Source: three-view drawing plus pictorial views. Frame: mm from the lowest corner of the part. Coordinates: 2 decimals unless noted, no trailing zeros. Write each loop counter-clockwise with the first axis right and the second up, starting at its lowest first coordinate (ties: lowest second). Pieces come first, ordered by that corner, then holes. Notation, with made-up numbers: (-21.5, 56.25) - (-11.5, 56.25) arc R23 ccw to (-11.5, 82.25) - close; hole circle Ø4 at (-22.75, 50.5). An arc over 180 degrees is marked (long way). One line per item, written item: value.
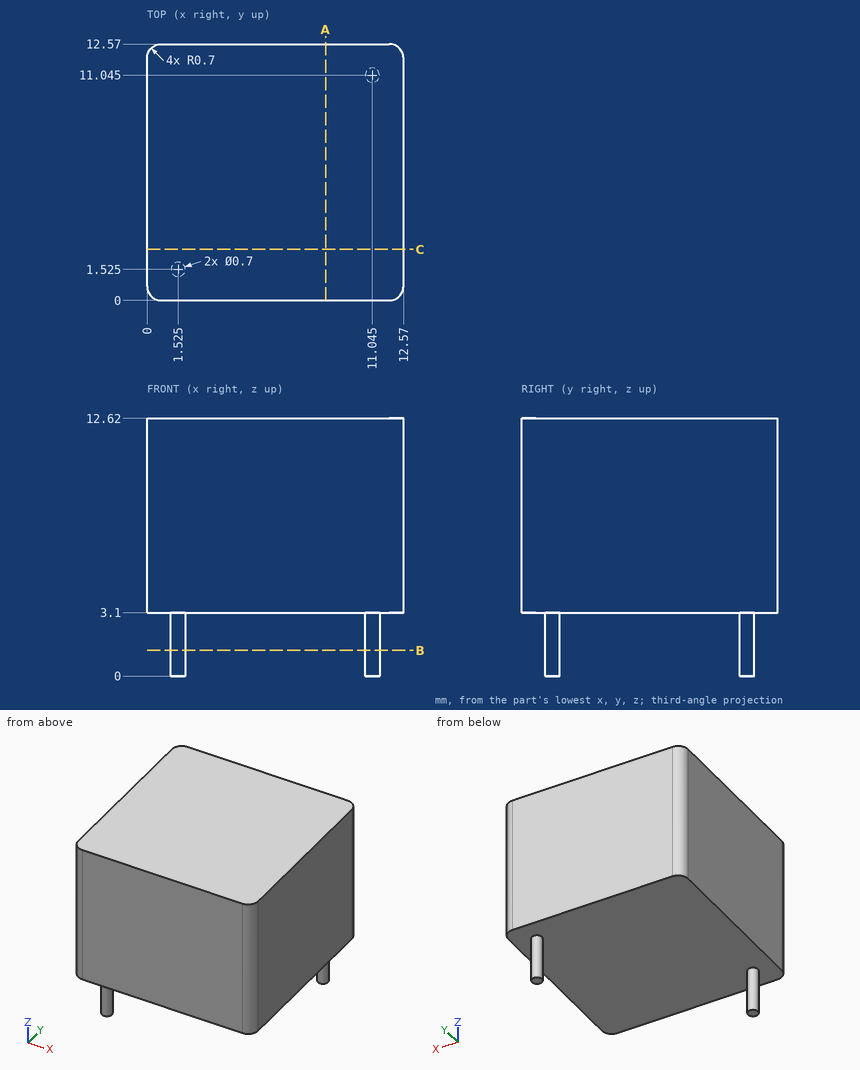
1) Section query B-B on z = 1.25. Output: boundary loops of the cut face in (x, y) (3 decimals), then the cut area to 3 significant figures.
Values found:
outline: circle Ø0.7 at (1.525, 1.525); circle Ø0.7 at (11.045, 11.045)
area: 0.770 mm2
2) Material intervals for line 1 (Z direction, x = 3.75, y = 10); line 2 (Y direction, x = 12, z = 11.5), sorted ascending.
Values found:
line 1: 3.1 to 12.62
line 2: 0.01 to 12.56
3) Contact query for flat-ended pins moving along their axis: P1, Ø4, axis at x = 5.5, z = 9.5, coming from the -Y side; P2, Ø5, axis at x = 5, y = 9, coming from the -Z side. Output: stop coordinate, or through.
Values found:
P1: y = 0
P2: z = 3.1
4) Section query A-A on x = 8.75. Output: boundary loops of the cut face in (y, z).
Values found:
outline: (0, 3.1) - (12.57, 3.1) - (12.57, 12.62) - (0, 12.62) - close
